Verification items for the finished model (mm, model axes). Face numbers are marked on the shaded views. A direction names the side the tool comes from. Give positions to 0.01 mm unless a question says otherwise; leave off trailing zeros. Order: outer loops, then holes, each group sorted by start corner. A loop starts at its lowest first (then second) coordinate and runs counter-clockwise, first axis right, second up. Notation, with made-up numbers: (50.5, -9) - (77.5, -9) arc R13 ccw to (77.5, 0) - close; hole circle Ø6 at (75.25, 68). An arc over 180 degrees is marked (long way). Answer as a JSON object with one key per item and string values. Group by question number.
(1) Mould release check, pull along X, two halves, no side actions. Record for the marked faces 3, 4 and 5: +X half, -X half, draft (parallel to the pull), parting line (faces both ways), or undercut.
(2) Depth check by flat-ended pin: pin 1 Ø1.5 at (x, y) = (-1, -12) entering from -Z; pin 2 Ø8 at (x, y) = (-5, -14) entering from -Z; pin 3 Ø1 at (y, z) = (-19, -0.5) entering from +X. Enter the tip coordinate at first touch or a pass-through.
(3) Section check B-B (z = 0). Record the boundary of the cut face in (x, y).
(4) Section check A-A (x = 0). Record the boundary of the cut face in (y, z).
(5) Thickness scan on line 1 (X direction, y = -4.25, z = 0); line 2 (Y direction, x = 1.25, z = -3.5); line 3 (Z direction, x = 2.5, y = -4). Record the ranges inside material, lowest first.
(6) Section check D-D (y = -14.5). Record the boundary of the cut face in (x, z).
(7) Access from +Z, -Z, +X, -X, +Y, -Y to the whole of each face (thin tool, end or side, straight path). Record for the marked faces 1 and 2.
(8) Section check C-C (y = -5). Record the boundary of the cut face in (x, z).
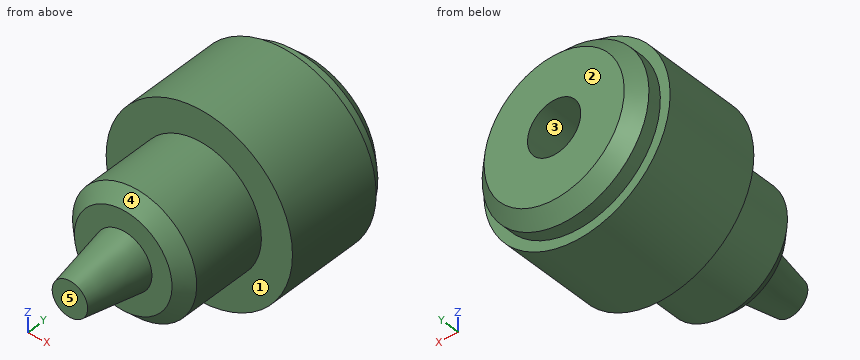
```python
from build123d import *

# Parameters (mm, degrees)
SKETCH_1_R          = 10.5
EXTRUDE_1_DEPTH     = 28
SKETCH_4_R          = 9.4
EXTRUDE_3_DEPTH     = 3
CHAMFER_2_SIZE      = 1.5
SKETCH_5_R          = 3
CUT_EXTRUDE_2_DEPTH = 14
CUT_EXTRUDE_START   = -17
SKETCH_6_R          = 10.5
SKETCH_6_R_2        = 7
CUT_EXTRUDE_3_DEPTH = 17
CUT_EXTRUDE_START_2 = -7
SKETCH_7_R          = 7
SKETCH_7_R_2        = 2
CUT_EXTRUDE_4_DEPTH = 7
CHAMFER_3_SIZE      = 1.5
DRAFT_3_ANGLE       = 10


with BuildPart() as part:
    # Эскиз1 → Бобышка-Вытянуть1 (new body)
    with BuildSketch(Plane(origin=(0, 0, 0), x_dir=(1, 0, 0), z_dir=(0, 1, 0))):
        with Locations(Location((0, 0, 0), (0, 0, 270))):
            Circle(SKETCH_1_R)
    extrude(amount=-EXTRUDE_1_DEPTH)

    # Эскиз4 → Бобышка-Вытянуть3 (add)
    with BuildSketch(Plane(origin=(0, 0, 0), x_dir=(1, 0, 0), z_dir=(0, 1, 0))):
        with Locations(Location((0, 0, 0), (0, 0, 270))):
            Circle(SKETCH_4_R)
    extrude(amount=EXTRUDE_3_DEPTH)

    # Фаска2
    chamfer_2_edges = [part.edges().sort_by_distance(p)[0] for p in [
        (0, 3, -9.4),
    ]]
    chamfer(chamfer_2_edges, length=CHAMFER_2_SIZE)

    # Эскиз5 → Вырез-Вытянуть2 (cut)
    with BuildSketch(Plane(origin=(0, 3, 0), x_dir=(1, 0, 0), z_dir=(0, 1, 0))):
        with Locations(Location((0, 0, 0), (0, 0, 270))):
            Circle(SKETCH_5_R)
    extrude(amount=-CUT_EXTRUDE_2_DEPTH, mode=Mode.SUBTRACT)

    # Эскиз6 → Вырез-Вытянуть3 (cut)
    with BuildSketch(Plane.XZ.offset(28).offset(CUT_EXTRUDE_START)):
        with Locations(Location((0, 0, 0), (0, 0, 90))):
            Circle(SKETCH_6_R)
        with Locations(Location((0, 0, 0), (0, 0, 270))):
            Circle(SKETCH_6_R_2, mode=Mode.SUBTRACT)
    extrude(amount=CUT_EXTRUDE_3_DEPTH, mode=Mode.SUBTRACT)

    # Эскиз7 → Вырез-Вытянуть4 (cut)
    with BuildSketch(Plane.XZ.offset(28).offset(CUT_EXTRUDE_START_2)):
        with Locations(Location((0, 0, 0), (0, 0, 270))):
            Circle(SKETCH_7_R)
        with Locations(Location((0, 0, 0), (0, 0, 270))):
            Circle(SKETCH_7_R_2, mode=Mode.SUBTRACT)
    extrude(amount=CUT_EXTRUDE_4_DEPTH, mode=Mode.SUBTRACT)

    # Фаска3
    chamfer_3_edges = [part.edges().sort_by_distance(p)[0] for p in [
        (0, -21, 7),
    ]]
    chamfer(chamfer_3_edges, length=CHAMFER_3_SIZE)

    # Уклон3
    draft_3_faces = [part.faces().sort_by_distance(p)[0] for p in [
        (0, -24.5, 2),
    ]]
    draft(draft_3_faces, Plane(origin=(0, -28, 0), x_dir=(0, 0, -1), z_dir=(0, -1, 0)), DRAFT_3_ANGLE)


solid = part.part
```
Solutions:
{
 "1": {"face 3": "undercut", "face 4": "parting line", "face 5": "draft"},
 "2": {"pin 1": "stops at z = -7", "pin 2": "stops at z = -10.23", "pin 3": "stops at x = 7"},
 "3": {"outline": "(-10.5, -11) - (-7, -11) - (-7, -19.5) - (-5.5, -21) - (-3.23, -21) - (-2, -28) - (2, -28) - (3.23, -21) - (5.5, -21) - (7, -19.5) - (7, -11) - (10.5, -11) - (10.5, 0) - (9.4, 0) - (9.4, 1.5) - (7.9, 3) - (3, 3) - (3, -11) - (-3, -11) - (-3, 3) - (-7.9, 3) - (-9.4, 1.5) - (-9.4, 0) - (-10.5, 0) - close"},
 "4": {"outline": "(-28, -2) - (-21, -3.23) - (-21, -5.5) - (-19.5, -7) - (-11, -7) - (-11, -10.5) - (0, -10.5) - (0, -9.4) - (1.5, -9.4) - (3, -7.9) - (3, -3) - (-11, -3) - (-11, 3) - (3, 3) - (3, 7.9) - (1.5, 9.4) - (0, 9.4) - (0, 10.5) - (-11, 10.5) - (-11, 7) - (-19.5, 7) - (-21, 5.5) - (-21, 3.23) - (-28, 2) - close"},
 "5": {"line 1": "x = -10.5 to -3, 3 to 10.5", "line 2": "y = -21 to 3", "line 3": "z = -10.2 to -1.66, 1.66 to 10.2"},
 "6": {"outline": "circle Ø14 at (0, 0)"},
 "7": {"face 1": "-Y", "face 2": "+Z, -Z, +X, -X, +Y"},
 "8": {"outline": "circle Ø21 at (0, 0); hole circle Ø6 at (0, 0)"}
}
